For this review, take the finished solid that the model builds, in its own axes (mm). A direction names the side the tool comes from. Coordinates: 2 decimals unless noted, no trailing zeros. Loops run counter-clockwise (first coordinate to the right, second up) from the corner with the lowest first, then second, coordinate; pieces in that order, holes last. Notation, with made-up numbers: (-12.75, 6.5) -> (44.25, 6.5) arc R24 cw to (44.25, 42.5) -> close; hole circle Ø1 at (32, 37). An arc over 180 degrees is marked (long way). Answer in a Markdown table with one row per item.
from build123d import *

# Parameters (mm, degrees)
EXTRUDE_1_DEPTH     = 6
CUT_EXTRUDE_1_DEPTH = 13.789155562
SKETCH_3_R          = 1.5
CUT_EXTRUDE_3_DEPTH = 16.692354826
FILLET_1_R          = 0.2


with BuildPart() as part:
    # ｽｹｯﾁ1 → ﾎﾞｽ - 押し出し1 (new body)
    with BuildSketch(Plane.XY):
        with BuildLine():
            Line((-5.25, -10), (-5.25, -1.064783644))
            Line((-5.25, -1.064783644), (-4.190017635, 1.641265431))
            ThreePointArc((-4.190017635, 1.641265431), (0, 4.5), (4.190017635, 1.641265431))
            Line((4.190017635, 1.641265431), (5.25, -1.064783644))
            Line((5.25, -1.064783644), (5.25, -10))
            Line((5.25, -10), (1.75, -10))
            Line((1.75, -10), (1.75, -2.185749299))
            ThreePointArc((1.75, -2.185749299), (0, 2.8), (-1.75, -2.185749299))
            Line((-1.75, -2.185749299), (-1.75, -10))
            Line((-1.75, -10), (-5.25, -10))
        make_face()
    extrude(amount=EXTRUDE_1_DEPTH)

    # ｽｹｯﾁ2 → ｶｯﾄ - 押し出し1 (cut, through all)
    with BuildSketch(Plane.XY.offset(6)):
        with BuildLine():
            Line((-5.25, -6.84287465), (-5.25, -5.34287465))
            ThreePointArc((-5.25, -5.34287465), (-5, -6.09287465), (-5.25, -6.84287465))
        make_face()
        with BuildLine():
            Line((5.25, -6.84287465), (5.25, -5.34287465))
            ThreePointArc((5.25, -5.34287465), (5, -6.09287465), (5.25, -6.84287465))
        make_face()
    extrude(amount=-CUT_EXTRUDE_1_DEPTH, mode=Mode.SUBTRACT)

    # ｽｹｯﾁ3 → ｶｯﾄ - 押し出し3 (cut, through all)
    with BuildSketch(Plane.ZY.offset(5.25)):
        with Locations(Location((3, -6.09287465, 0), (0, 0, 330))):
            Circle(SKETCH_3_R)
    extrude(amount=-CUT_EXTRUDE_3_DEPTH, mode=Mode.SUBTRACT)

    # ﾌｨﾚｯﾄ1
    fillet_1_edges = [part.edges().sort_by_distance(p)[0] for p in [
        (1.75, -2.185749299, 3),
        (-1.75, -2.185749299, 3),
        (-1.75, -10, 3),
        (-5.25, -10, 3),
        (5.25, -10, 3),
        (1.75, -10, 3),
    ]]
    fillet(fillet_1_edges, radius=FILLET_1_R)


solid = part.part
Item 1: Insertion check: pin 1 (1 mm diameter, centred on x = -1, z = 3.5, fed in from +Y); pin 2 (1.8 mm diameter, centred on y = -6.09, z = 3, fed in from -X); pin 3 (1 mm diameter, centred on x = 2, z = 2, fed in from +Y). Each pin has a flat end and moves straight along its axis. Give the tip position at first contact, or say it passes through.
Worked answers:
| item | result |
|---|---|
| pin 1 | y = 4.47 |
| pin 2 | through |
| pin 3 | y = 4.24 |
Item 2: Take a section at A-A, the plane y = -3. State the section outline as (x, z) points.
Worked answers:
| item | result |
|---|---|
| outline | (-5.25, 0) -> (-1.75, 0) -> (-1.75, 6) -> (-5.25, 6) -> close; (1.75, 0) -> (5.25, 0) -> (5.25, 6) -> (1.75, 6) -> close |
Item 3: The part is to be moulded in two halves that separate along Z. For faces 3 (the flat face through (-5.25, -3, 3)), 4 (the flat face through (-2, -3, 6)), 5 (the cylindrical face through (-3.524, -4.707, 3.575)), say which applies: +Z half, -Z half, draft (parallel to the pull), parting line (faces both ways), or undercut.
Worked answers:
| item | result |
|---|---|
| face 3 | draft |
| face 4 | +Z half |
| face 5 | undercut |
Item 4: Take a section at C-C, the plane y = -6. State the section outline as (x, z) points.
Worked answers:
| item | result |
|---|---|
| outline | (-5, 0) -> (-1.75, 0) -> (-1.75, 1.5) -> (-5, 1.5) -> close; (-5, 4.5) -> (-1.75, 4.5) -> (-1.75, 6) -> (-5, 6) -> close; (1.75, 0) -> (5, 0) -> (5, 1.5) -> (1.75, 1.5) -> close; (1.75, 4.5) -> (5, 4.5) -> (5, 6) -> (1.75, 6) -> close |
Item 5: Take a section at B-B, the plane z = 3. State the section outline as (x, y) points, and give its area (3 significant figures).
Worked answers:
| item | result |
|---|---|
| outline | (-5.25, -9.8) arc R0.2 ccw to (-5.05, -10) -> (-1.95, -10) arc R0.2 ccw to (-1.75, -9.8) -> (-1.75, -7.59) -> (-5.25, -7.59) -> close; (-5.25, -4.59) -> (-1.75, -4.59) -> (-1.75, -2.28) arc R0.2 ccw to (-1.82, -2.13) arc R2.8 cw (long way) to (1.82, -2.13) arc R0.2 ccw to (1.75, -2.28) -> (1.75, -4.59) -> (5.25, -4.59) -> (5.25, -1.06) -> (4.19, 1.64) arc R4.5 ccw to (-4.19, 1.64) -> (-5.25, -1.06) -> close; (1.75, -9.8) arc R0.2 ccw to (1.95, -10) -> (5.05, -10) arc R0.2 ccw to (5.25, -9.8) -> (5.25, -7.59) -> (1.75, -7.59) -> close |
| area | 65.2 mm² |
Item 6: Take a section at D-D, the plane z = 5. State the section outline as (x, y) points, and give its area (3 significant figures).
Worked answers:
| item | result |
|---|---|
| outline | (-5.25, -9.8) arc R0.2 ccw to (-5.05, -10) -> (-1.95, -10) arc R0.2 ccw to (-1.75, -9.8) -> (-1.75, -2.28) arc R0.2 ccw to (-1.82, -2.13) arc R2.8 cw (long way) to (1.82, -2.13) arc R0.2 ccw to (1.75, -2.28) -> (1.75, -9.8) arc R0.2 ccw to (1.95, -10) -> (5.05, -10) arc R0.2 ccw to (5.25, -9.8) -> (5.25, -6.84) arc R1.25 cw to (5.25, -5.34) -> (5.25, -1.06) -> (4.19, 1.64) arc R4.5 ccw to (-4.19, 1.64) -> (-5.25, -1.06) -> (-5.25, -5.34) arc R1.25 cw to (-5.25, -6.84) -> close |
| area | 85.7 mm² |
Item 7: For L1, parallel to X at y = -9.25, z = 5; L2, parallel to Y at x = -2.25, z = 4.25; L3, parallel to X at y = 0, z = 2.6, list the stretches that pass through material, from the lowest coordinate up.
Worked answers:
| item | result |
|---|---|
| L1 | -5.25 to -1.75, 1.75 to 5.25 |
| L2 | -10 to -6.92, -5.26 to -1.67, 1.67 to 3.9 |
| L3 | -4.83 to -2.8, 2.8 to 4.83 |
Item 8: For faces 1 (the flat face through (-1.75, -5.2, 1.6)), 2 (the flat face through (4, -10, 3)), list the 3-axis set-ups (+Z, -Z, +X, -X, +Y, -Y) from which the entire face can be reached by the end or side of a thin tool; tool diameter is ignored.
Worked answers:
| item | result |
|---|---|
| face 1 | +Z, -Z, -Y |
| face 2 | +Z, -Z, +X, -X, -Y |
